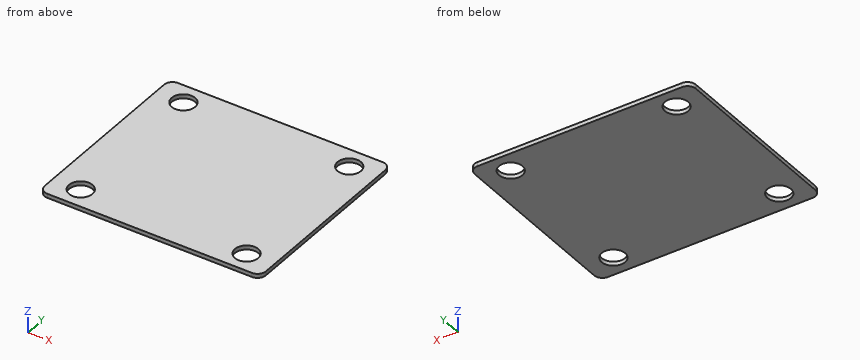
Autodesk Inventor part; units mm, degrees
ref_plane "YZ Plane" through (0, 0, 0) normal (1, 0, 0) x (0, 1, 0)
ref_plane "XZ Plane" through (0, 0, 0) normal (0, 1, 0) x (-1, 0, 0)
ref_plane "XY Plane" through (0, 0, 0) normal (0, 0, 1) x (1, 0, 0)
sketch3d "3D Sketch1"
sketch "Sketch1" plane through (0, 0, 0) normal (0, 0, 1) x (1, 0, 0)
  line L0 (-56, 70) -> (56, 70)
  line L1 (56, 70) -> (56, -70) construction
  line L2 (56, -70) -> (-56, -70)
  line L3 (-56, -70) -> (-56, 70) construction
  line L4 (-56, 70) -> (56, -70) construction
  line L5 (56, 70) -> (-56, -70) construction
  line L6 (56, -70) -> (80, -70)
  line L7 (80, -70) -> (80, 70)
  line L8 (80, 70) -> (56, 70)
  line L9 (-56, -70) -> (-80, -70)
  line L10 (-80, -70) -> (-80, 70)
  line L11 (-80, 70) -> (-56, 70)
  circle A0 centre (60, -55) radius 8.5
  circle A1 centre (60, 55) radius 8.5
  circle A2 centre (-60, -55) radius 8.5
  circle A3 centre (-60, 55) radius 8.5
  line L12 (0, -70) -> (0, 70) construction
  line L13 (80, 0) -> (-80, 0) construction
  point P0 (0, 0)
  dimension "d30" = 140
  dimension "d34" = 160
  dimension "d35" = 17
  dimension "d36" = 20
  dimension "d37" = 15
extrude "Plate1" add sketch "Sketch1" along normal blind 3
fillet "Corner Round1" radius 6 4 edges at (80, 70, 1.5) (-80, 70, 1.5) (-80, -70, 1.5) (80, -70, 1.5)
equation "\"d6\" = Thickness"
equation "\"BendReliefWidth\" = Thickness"
equation "\"BendReliefDepth\" = 0.5 * Thickness"
equation "\"CornerReliefSize\" = 4 * Thickness"
equation "\"MinimumRemnant\" = 2 * Thickness"
equation "\"TransitionRadius\" = BendRadius"
equation "\"JacobiRadiusSize\" = BendRadius"
equation "\"GapSize\" = Thickness"
properties part number "MSC 081 pillar 1" material "Stainless Steel"
Geometry: final body of the model. Coordinates: model frame, mm. Coordinates: 2 decimals unless noted, no trailing zeros. Order: outer loops, then holes, each group sorted by start corner. A loop starts at its lowest first (then second) coordinate and runs counter-clockwise, first axis right, second up. Notation, with made-up numbers: (66, -24) -> (118, -24) arc R29 ccw to (118, 2) -> close; hole circle Ø9 at (35.5, 61). An arc over 180 degrees is marked (long way). Write item = value, one per line.
(1) Cut plane A-A on y = -55. Return loops of the section in (x, z).
Solved:
outline = (-80, 0) -> (-68.5, 0) -> (-68.5, 3) -> (-80, 3) -> close; (-51.5, 0) -> (51.5, 0) -> (51.5, 3) -> (-51.5, 3) -> close; (68.5, 0) -> (80, 0) -> (80, 3) -> (68.5, 3) -> close
(2) Line query: line 1 (Y direction, x = -60, z = 1); line 2 (X direction, y = 48, z = 1). Output: solid intervals per line, ascending.
Solved:
line_1 = -70 to -63.5, -46.5 to 46.5, 63.5 to 70
line_2 = -80 to -64.82, -55.18 to 55.18, 64.82 to 80
(3) Cut plane B-B on x = -60. Return loops of the section in (y, z), plus the area to 3 significant figures.
Solved:
outline = (-70, 0) -> (-63.5, 0) -> (-63.5, 3) -> (-70, 3) -> close; (-46.5, 0) -> (46.5, 0) -> (46.5, 3) -> (-46.5, 3) -> close; (63.5, 0) -> (70, 0) -> (70, 3) -> (63.5, 3) -> close
area = 318 mm²
(4) Pin query (flat end, axial travel): pin 1 Ø1.5 at (x, y) = (-21.5, -2.5) entering from -Z. Return the tip coordinate at first contact, or that it passes through.
Solved:
pin_1 = 0
(5) Cut plane C-C on z = 2.25. Return loops of the section in (x, y).
Solved:
outline = (-80, -64) arc R6 ccw to (-74, -70) -> (74, -70) arc R6 ccw to (80, -64) -> (80, 64) arc R6 ccw to (74, 70) -> (-74, 70) arc R6 ccw to (-80, 64) -> close; hole circle Ø17 at (-60, -55); hole circle Ø17 at (-60, 55); hole circle Ø17 at (60, -55); hole circle Ø17 at (60, 55)
